```python
from build123d import *

# Parameters (mm, degrees)
SKETCH_1_R          = 50
EXTRUDE_1_DEPTH     = 10
FILLET_1_R          = 20
FILLET_2_R          = 35
CUT_EXTRUDE_START   = -12
CUT_EXTRUDE_1_DEPTH = 12
FILLET_3_R          = 5


with BuildPart() as part:
    # 草图1 → 凸台-拉伸1 (new body)
    with BuildSketch(Plane(origin=(0, 0, 0), x_dir=(0, 0, -1), z_dir=(1, 0, 0))):
        with BuildLine():
            Line((-212, -91), (-50, -91))
            Line((-50, -91), (23.592526884, -63.776113673))
            ThreePointArc((23.592526884, -63.776113673), (67.999915285, -0.107337145), (23.793748654, 63.701314939))
            Line((23.793748654, 63.701314939), (-60, 95))
            Line((-60, 95), (-76.255769572, 95))
            ThreePointArc((-76.255769572, 95), (-105.931697447, 32.698838939), (-170.519226707, 57))
            Line((-170.519226707, 57), (-212, 57))
            Line((-212, 57), (-212, -6))
            Line((-212, -6), (-150, -6))
            ThreePointArc((-150, -6), (-130, -26), (-150, -46))
            Line((-150, -46), (-212, -46))
            Line((-212, -46), (-212, -91))
        make_face()
        Circle(SKETCH_1_R, mode=Mode.SUBTRACT)
    extrude(amount=EXTRUDE_1_DEPTH)

    # 圆角1
    fillet_1_edges = [part.edges().sort_by_distance(p)[0] for p in [
        (5, 57, 212),
        (5, -91, 212),
    ]]
    fillet(fillet_1_edges, radius=FILLET_1_R)

    # 圆角2
    fillet_2_edges = [part.edges().sort_by_distance(p)[0] for p in [
        (5, -6, 212),
    ]]
    fillet(fillet_2_edges, radius=FILLET_2_R)

    # 草图2 → 切除-拉伸1 (cut)
    with BuildSketch(Plane(origin=(10, 0, 0), x_dir=(0, 0, -1), z_dir=(1, 0, 0)).offset(CUT_EXTRUDE_START)):
        with BuildLine():
            Line((-42.462460206, 26.399611233), (-51.481550921, 25.61054304))
            ThreePointArc((-51.481550921, 25.61054304), (-57.28119514, -5.011455208), (-46.252206356, -34.161138845))
            Line((-46.252206356, -34.161138845), (-37.233115641, -33.372070653))
            ThreePointArc((-37.233115641, -33.372070653), (-49.809734905, -4.357787137), (-42.462460206, 26.399611233))
        make_face()
    extrude(amount=CUT_EXTRUDE_1_DEPTH, mode=Mode.SUBTRACT)

    # 圆角3
    fillet_3_edges = [part.edges().sort_by_distance(p)[0] for p in [
        (5, -34.161138845, 46.252206356),
        (5, 25.61054304, 51.481550921),
    ]]
    fillet(fillet_3_edges, radius=FILLET_3_R)


solid = part.part
```
Could you check a few things on this model? Use its own coordinates, in mm. A direction names the side the tool comes from. Coordinates: 2 decimals unless noted, no trailing zeros. Loops run counter-clockwise (first coordinate to the right, second up) from the corner with the lowest first, then second, coordinate; pieces in that order, holes last. Notation, with made-up numbers: M 76,32 L 91,32 A25 ccw 91,69 Z; hole C 34.5,32 d8. An arc over 180 degrees is marked long. Put each result on its own line as item: value. Start each with the question number.
(1) Suppose I cut it at B-B on x = 4.5. Please give me the cut outline in (y, z), then the cut area to 3 significant figures.
(2) Suppose I cut it at C-C on y = 0. Please give me the cut outline in (x, z), then the cut area to 3 significant figures.
(3) I need wall thicknesses on line 1 (Z direction, x = 5, y = 0); line 2 (Y direction, x = 5, z = -38); line 3 (Y direction, x = 2, z = 0). Which ranges of each line are inside material? Lowest first, please. Write a range as from..to.
(4) Thinking about a two-plate mould opening in Y: for faces 1 (the face through (5, -58, 212)), 2 (the face through (5.07, 3.981, 201.475)), 3 (the face through (4.93, -77.58, 13.72)), which applies, pulls with the +Y half, pulls with the -Y half, needs draft (parallel to the pull), parting line crosses it, or undercut?
(5) Suppose I cut it at A-A on z = 0. Please give me the cut outline in (x, y).
(6) For faces 4 (the face through (4.93, -4.613, 57.315)), 5 (the face through (5, -46, 181)), 6 (the face through (5, 57, 181)), 7 (the face through (0, -17, 74)), which set-ups out of +Z, -Z, +X, -X, +Y, -Y let a thin tool reach every point of the face, with its end or its side?
(7) Will these pins go through, and if not, where does the flat tip stop? P1, Ø2, axis at x = 1.5, z = 111.5, coming from the +Y side; P2, Ø4, axis at x = 8.5, y = 64, coming from the +Z side; P3, Ø1.5, axis at x = 5.5, y = 33.5, coming from the -Z side.
(8) Suppose I cut it at D-D on z = 83.5. Please give me the cut outline in (x, y), then the cut area to 3 significant figures.
Solutions:
1. outline: M -91,50 L -63.78,-23.59 A68 ccw 63.7,-23.79 L 95,60 L 95,76.26 A51 cw 57,170.52 L 57,192 A20 ccw 37,212 L 29,212 A35 ccw -6,177 L -6,150 A20 cw -46,150 L -46,212 L -71,212 A20 ccw -91,192 Z; hole M -33.91,43.38 L -33.37,37.23 A50 ccw long 26.4,42.46 L 25.86,48.6 A5 ccw 22.87,52.76 A57.5 ccw -31.68,47.98 A5 ccw Z
1. area: 26,700 mm2
2. outline: M 0,-68 L 10,-68 L 10,-50 L 0,-50 Z; M 0,57.5 L 10,57.5 L 10,196.6 L 0,196.6 Z
2. area: 1,570 mm2
3. line 1: z = -68..-50, 57.5..196.6
3. line 2: y = -56.39..-32.5, 32.5..56.39
3. line 3: y = -72.5..-50, 50..72.59
4. face 1: needs draft
4. face 2: undercut
4. face 3: pulls with the -Y half
5. outline: M 0,-72.5 L 10,-72.5 L 10,-50 L 0,-50 Z; M 0,50 L 10,50 L 10,72.59 L 0,72.59 Z
6. face 4: +X, -X
6. face 5: +Z, +X, -X
6. face 6: +Z, +X, -X, +Y
6. face 7: +Z, -Z, -X, +Y, -Y
7. P1: stops at y = 31.1
7. P2: stops at z = 77.28
7. P3: stops at z = -59.59
8. outline: M 0,-91 L 10,-91 L 10,50.36 L 0,50.36 Z
8. area: 1,410 mm2
